Source: CAD feature listing. Evaluate the final solid. Frame: model axes, mm. Face numbers are marked on the shaded views. A direction names the side the tool comes from. Round coordinates to 2 decimals unless told otherwise and drop trailing zeros. Loops run counter-clockwise (first coordinate to the right, second up) from the corner with the lowest first, then second, coordinate; pieces in that order, holes last.
(1) Section D-D, the plane y = 7.75. Return the cut outline in (x, z), plus the area to 3 significant figures.
(2) Section C-C, the plane x = 48. Return the cut outline in (y, z), plus the area to 3 significant figures.
(3) Material intervals for probe 1 along Y at (x, z) = (8.5, -2.25); probe 2 along Y at (x, z) = (50, -2); probe 3 along Z at (x, y) = (3.5, 1.1), sorted ascending.
(4) Section B-B, the plane z = -3.25. Return the cut outline in (x, y), plus the area to 3 significant figures.
(5) Mould query, pull axis Y, two halves, no side actions, for the marked faces 1, 2, 3 and 4. Classes: pulls with the +Y half, pulls with the -Y half, needs draft (parallel to the pull), parting line crosses it, or undercut.
(6) Section A-A, the plane x = 8. Return the cut outline in (y, z).
(7) Set-up query: the marked faces 5, 6 and 7. Return all of +Z, -Z, +X, -X, +Y, -Y with unobstructed straight access to the full face (end or side cutting, diameter ignored); none if empty.
(8) First-contact query: pin 1 Ø1.6 at (y, z) = (10, 0) entering from -X; pin 2 Ø4 at (y, z) = (7.5, -0.5) entering from -X; pin 3 Ø5 at (x, z) = (44, -0.5) entering from -Y; pin 4 Ø2 at (x, z) = (3.5, 0) entering from +Y. Flat tips, straight axial feed; report the tip coordinate or a pass-through.
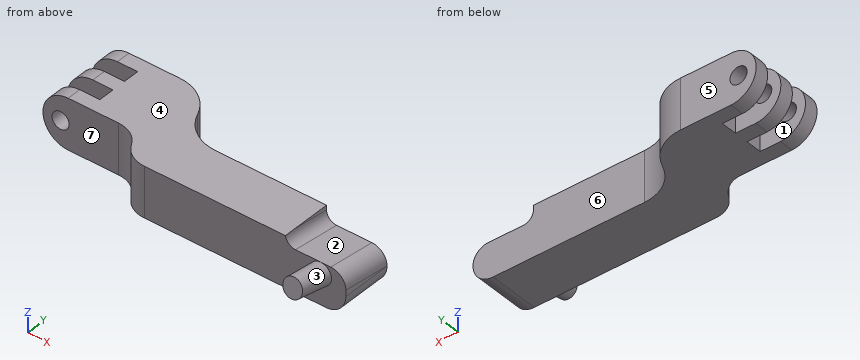
```python
from build123d import *

# Parameters (mm, degrees)
PAD008_DEPTH    = 5
POCKET013_DEPTH = 20.801
SKETCH027_R     = 1.7
POCKET014_DEPTH = 14.801
POCKET015_DEPTH = 12
FILLET007_R     = 3
FILLET008_R     = 2
FILLET009_R     = 4


with BuildPart() as part:
    # Sketch025 → Pad008 (new body, symmetric)
    with BuildSketch(Plane.XY):
        with BuildLine():
            Line((0, 0), (0, 2.8))
            Line((0, 2.8), (9, 2.8))
            Line((9, 2.8), (9, 6))
            Line((9, 6), (0, 6))
            Line((0, 6), (0, 8.8))
            Line((0, 8.8), (9, 8.8))
            Line((9, 8.8), (9, 12))
            Line((9, 12), (0, 12))
            Line((0, 12), (0, 14.8))
            Line((0, 14.8), (9, 14.8))
            Line((9, 14.8), (15, 14.8))
            ThreePointArc((23, 9.4), (19.8259714048, 13.3236613405), (15, 14.8))
            ThreePointArc((23, 9.4), (26.1740285952, 5.4763386595), (31, 4))
            Line((31, 4), (65, 4))
            Line((65, 4), (65, -6))
            Line((25, -6), (65, -6))
            ThreePointArc((20, -3), (22.0845240526, -5.1924599124), (25, -6))
            ThreePointArc((20, -3), (17.9154759474, -0.8075400876), (15, 0))
            Line((15, 0), (0, 0))
        make_face()
    extrude(amount=PAD008_DEPTH, both=True)

    # Sketch026 (on Face18 of Pad008) → Pocket013 (cut, through all)
    with BuildSketch(Plane.XZ.offset(6)):
        with BuildLine():
            ThreePointArc((5, 5), (0, 0), (5, -5))
            Line((5, -6), (5, -5))
            Line((-1, -6), (5, -6))
            Line((-1, 6), (-1, -6))
            Line((5, 6), (-1, 6))
            Line((5, 6), (5, 5))
        make_face()
    extrude(amount=-POCKET013_DEPTH, mode=Mode.SUBTRACT)

    # Sketch027 (on Face3 of Pocket013) → Pocket014 (cut, through all)
    with BuildSketch(Plane.XZ):
        with Locations((3.5, 0)):
            Circle(SKETCH027_R)
    extrude(amount=-POCKET014_DEPTH, mode=Mode.SUBTRACT)

    # Sketch028 (on DatumLine) → Revolution001 (revolve)
    with BuildSketch(Plane(origin=(60, 0, 0), x_dir=(0, -0.1736481777, -0.984807753), z_dir=(1, 0, 0))):
        Polygon((0, -5), (2.1902294727, -5), (1.95, -13), (0, -13), align=None)
    revolve(axis=Axis((60, 0, 0), (0, 0.984807753, -0.1736481777)))

    # Sketch029 (on Face23 of Revolution001) → Pocket015 (cut)
    with BuildSketch(Plane.YZ.offset(65)):
        Polygon((-6, 3.25), (6, 1.8615526279), (6, 6.8615526279), (-6, 6.8615526279), align=None)
    extrude(amount=-POCKET015_DEPTH, mode=Mode.SUBTRACT)

    # Fillet007
    fillet007_edges = [part.edges().sort_by_distance(p)[0] for p in [
        (65, -1, 2.67148),
    ]]
    fillet(fillet007_edges, radius=FILLET007_R)

    # Fillet008
    fillet008_edges = [part.edges().sort_by_distance(p)[0] for p in [
        (53, -1, 2.67148),
    ]]
    fillet(fillet008_edges, radius=FILLET008_R)

    # Fillet009
    fillet009_edges = [part.edges().sort_by_distance(p)[0] for p in [
        (65, -1, -5),
    ]]
    fillet(fillet009_edges, radius=FILLET009_R)


solid = part.part
```
Output values:
1. outline: (5, -5) - (23.88, -5) - (23.88, 5) - (5, 5) arc R5 ccw to start; hole circle Ø3.4 at (3.5, 0)
1. area: 219 mm2
2. outline: (-6, -5) - (4, -5) - (4, 5) - (-6, 5) - close
2. area: 100 mm2
3. probe 1: y = 0 to 2.8, 6 to 8.8, 12 to 14.8
3. probe 2: y = -6 to 4
3. probe 3: z = -4.77 to -1.7, 1.7 to 4.77
4. outline: (1.2, 0) - (15, 0) arc R5.67 cw to (20, -3) arc R5.67 ccw to (25, -6) - (64.31, -6) - (64.31, 4) - (31, 4) arc R8.63 cw to (23, 9.4) arc R8.63 ccw to (15, 14.8) - (1.2, 14.8) - (1.2, 12) - (9, 12) - (9, 8.8) - (1.2, 8.8) - (1.2, 6) - (9, 6) - (9, 2.8) - (1.2, 2.8) - close
4. area: 704 mm2
5. face 1: undercut
5. face 2: pulls with the +Y half
5. face 3: undercut
5. face 4: needs draft
6. outline: (0, -5) - (2.8, -5) - (2.8, 5) - (0, 5) - close; (6, -5) - (8.8, -5) - (8.8, 5) - (6, 5) - close; (12, -5) - (14.8, -5) - (14.8, 5) - (12, 5) - close
7. face 5: +Z, -Z, +X, -X, +Y
7. face 6: +Z, -Z, +X, +Y
7. face 7: +Z, -Z, -X, -Y
8. pin 1: stops at x = 9
8. pin 2: stops at x = 0
8. pin 3: stops at y = -6
8. pin 4: passes through
